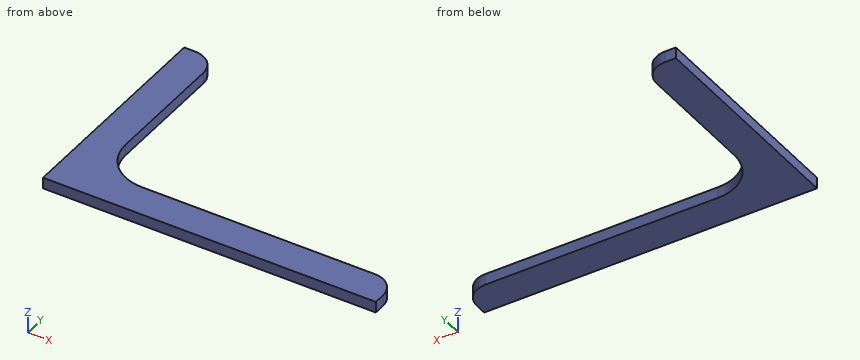
Autodesk Inventor part; units mm, degrees
ref_plane "Начальная плоскость" through (0, 0, 0) normal (0, 0, 1) x (1, 0, 0)
ref_plane "Конечная плоскость" through (0, 0, 1) normal (0, 0, 1) x (1, 0, 0)
ref_plane "YZ Plane" through (0, 0, 0) normal (1, 0, 0) x (0, 1, 0)
ref_plane "Начальная плоскость" through (0, 0, 0) normal (0, 0, 1) x (1, 0, 0)
ref_plane "Конечная плоскость" through (0, 0, 1) normal (0, 0, 1) x (1, 0, 0)
sketch "Эскиз" plane through (0, 0, 0) normal (0, 0, 1) x (1, 0, 0)
  line L0 (-6.9, 1.98) -> (-6.9, 12.98)
  line L1 (-9.9, 14.98) -> (-8.9, 14.98)
  line L2 (-9.9, -5.02) -> (-9.9, 14.98)
  line L3 (-9.9, -5.02) -> (20.1, -5.02)
  line L4 (20.1, -4.02) -> (20.1, -5.02)
  line L5 (-2.9, -2.02) -> (18.1, -2.02)
  arc A0 (-6.9, 1.98) -> (-2.9, -2.02) centre (-2.9, 1.98) ccw
  arc A1 (-6.9, 12.98) -> (-8.9, 14.98) centre (-8.9, 12.98) ccw
  arc A2 (20.1, -4.02) -> (18.1, -2.02) centre (18.1, -4.02) ccw
  line L6 (20.1, 0) -> (-9.9, 0) construction
  line L7 (0, -5.02) -> (0, 14.98) construction
  line L8 (0, 0) -> (30, 0) construction
  point P0 (-6.9, -2.02)
  point P1 (-6.9, 14.98)
  point P2 (20.1, -2.02)
  dimension "d17" = 4
  dimension "d19" = 2
  dimension "d26" = 5.02
  dimension "d27" = 9.9
  dimension "d28" = 20
  dimension "d29" = 30
  dimension "d30" = 3
  dimension "d31" = 3
  dimension "d32" = 90
extrude "Базовый элемент" add sketch "Эскиз" along normal up to surface (1 mm away) from surface at 0
sketch "Sketch3" plane through (0, 0, 0) normal (0, 0, 1) x (1, 0, 0)
  line L0 (0, 0) -> (10, 0)
ref_plane "Work Plane10" through (0, 0, 0) normal (0, -1, 0) x (1, 0, 0)
sketch "Sketch4" plane through (0, 0, 0) normal (0, -1, 0) x (1, 0, 0)
  line L0 (-2, 0) -> (12, 0)
  line L1 (-2, 1) -> (12, 1)
  dimension "d25" = 1
equation "\"d17\" = R"
equation "\"d19\" = R1"
equation "\"d26\" = ey"
equation "\"d27\" = ex"
equation "\"d28\" = b"
equation "\"d29\" = ParH"
equation "\"d30\" = ParT"
equation "\"d31\" = ParT"
equation "\"d11\" = G_L"
equation "\"b\" = 20"
equation "\"ParT\" = 3"
equation "\"R\" = 4"
equation "\"G_L\" = d25"
equation "\"R1\" = 2"
equation "\"G_OFFSET_START\" = 0"
equation "\"G_OFFSET_END\" = 0"
equation "\"d21\" = G_OFFSET_END + B_L"
equation "\"ex\" = 9.9"
equation "\"ey\" = 5.02"
equation "\"B_L\" = 1"
equation "\"ParH\" = 30"
properties part number "Кутик ДСТУ 2251" material "С245 ДСТУ 8539"
Model file for the job. Use its own axes, mm. Give positions to 0.01 mm unless a question says otherwise; leave off trailing zeros. Loops run counter-clockwise (first coordinate to the right, second up) from the corner with the lowest first, then second, coordinate; pieces in that order, holes last. Notation, with made-up numbers: (-7, 75.25) -> (35, 75.25) arc R18 ccw to (35, 84.25) -> close; hole circle Ø2 at (32, 37.5). An arc over 180 degrees is marked (long way). Use a Markdown table: item, result. Add a question column.
(1) Slice it at B-B on x = 15. List the corners of the cut face in (y, z).
(2) Slice it at A-A on z = 0.55. List the corners of the cut face in (x, y).
(3) Slice it at C-C on y = 5.75. List the corners of the cut face in (x, z), and give its area (3 significant figures).
(4) Wall check: line 1 along Y through (x, z) = (6, 0.65); line 2 along X through (y, z) = (8.5, 0.95); line 3 along X through (y, z) = (1, 0.9). Give the ranges that are in metal, low to high.
Filled sheet:
| question | item | result |
|---|---|---|
| 1 | outline | (-5.02, 0) -> (-2.02, 0) -> (-2.02, 1) -> (-5.02, 1) -> close |
| 2 | outline | (-9.9, -5.02) -> (20.1, -5.02) -> (20.1, -4.02) arc R2 ccw to (18.1, -2.02) -> (-2.9, -2.02) arc R4 cw to (-6.9, 1.98) -> (-6.9, 12.98) arc R2 ccw to (-8.9, 14.98) -> (-9.9, 14.98) -> close |
| 3 | outline | (-9.9, 0) -> (-6.9, 0) -> (-6.9, 1) -> (-9.9, 1) -> close |
| 3 | area | 3.00 mm2 |
| 4 | line 1 | -5.02 to -2.02 |
| 4 | line 2 | -9.9 to -6.9 |
| 4 | line 3 | -9.9 to -6.78 |
